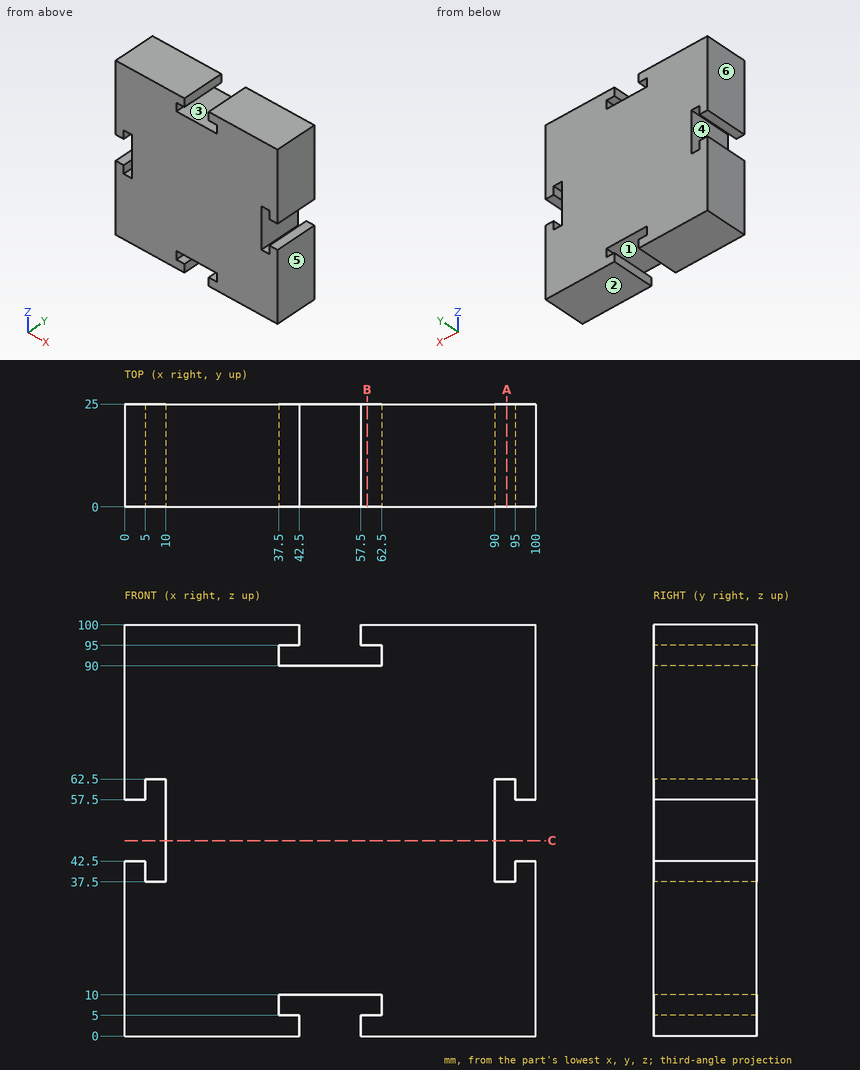
Verification items for this drawing (mm, ordinates from the low corner). A direction names the side the tool comes from. Give positions to 0.01 mm unless a question says otherwise; leave off trailing zeros. Loops run counter-clockwise (first coordinate to the right, second up) from the corner with the lowest first, then second, coordinate; pieces in that order, holes last.
1. Material ranges on probe 1 along X at (y, z) = (6.25, 40); probe 2 along Z at (x, y) = (95.5, 5), recorded low to high.
Derived:
probe 1: x = 0 to 5, 10 to 90, 95 to 100
probe 2: z = 0 to 42.5, 57.5 to 100
2. Cross-section at A-A on x = 93. Record the cut outline in (y, z), and give its area (4 significant figures).
Derived:
outline: (0, 0) - (25, 0) - (25, 37.5) - (0, 37.5) - close; (0, 62.5) - (25, 62.5) - (25, 100) - (0, 100) - close
area: 1,875 mm2
3. Release check for a two-part mould opening along X. For the marked faces 3, 4, 5 and 6 record: +X half, -X half, draft (parallel to the pull), parting line (faces both ways), or undercut.
Derived:
face 3: undercut
face 4: undercut
face 5: +X half
face 6: -X half
4. Cross-section at B-B on x = 59. Record the cut outline in (y, z), and give its area (3 significant figures).
Derived:
outline: (0, 0) - (25, 0) - (25, 5) - (0, 5) - close; (0, 10) - (25, 10) - (25, 90) - (0, 90) - close; (0, 95) - (25, 95) - (25, 100) - (0, 100) - close
area: 2,250 mm2
5. Cross-section at C-C on z = 47.5. Record the cut outline in (x, y).
Derived:
outline: (10, 0) - (90, 0) - (90, 25) - (10, 25) - close
6. Tool access check on the marked faces 1 and 2. Record the directions out of +Z, -Z, +X, -X, +Y, -Y that give a thin tool (end or side, any length) a straight path to the whole face; none if there is none.
Derived:
face 1: +Y, -Y
face 2: -Z, +X, -X, +Y, -Y
